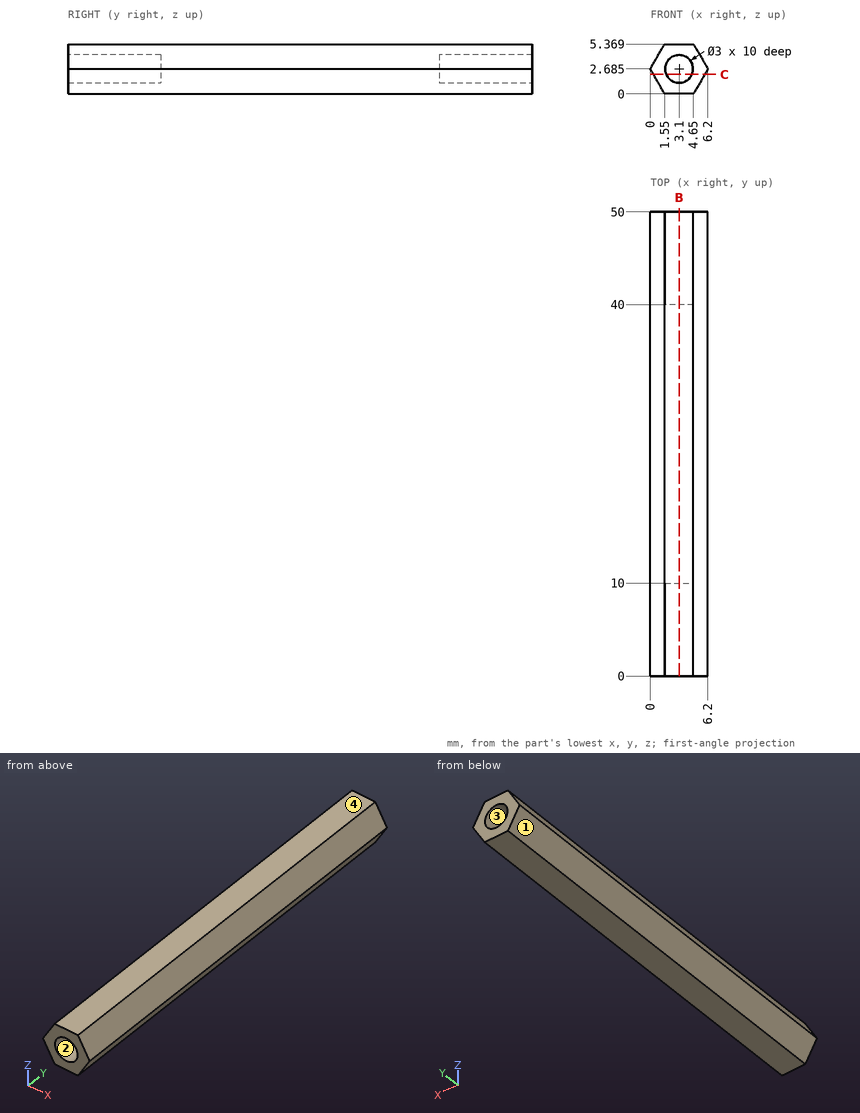
Geometry: see drawing. Coordinates: mm, zero at the bounding-box minimum. Give positions to 0.01 mm unless a question says otherwise; leave off trailing zeros. Loops run counter-clockwise (first coordinate to the right, second up) from the corner with the lowest first, then second, coordinate; pieces in that order, holes last. Notation, with made-up numbers: (58, 28) -> (72, 28) arc R9 ccw to (72, 35) -> close; hole circle Ø2 at (42.25, 34.5). An arc over 180 degrees is marked (long way). Answer as a JSON object with one key per item and string values. Group by question number.
Item 1: Pin query (flat end, axial travel): P1, Ø2, axis at y = 6.5, z = 0.5, coming from the +X side. Return the tip coordinate at first contact, or that it passes through.
Item 2: Pull-direction query (X, two-part tool) for the marked faces 1, 2, 3 and 4; classes: released by +X, released by -X, zero draft, split by the parting line, or undercut.
Item 3: Line query: probe 1 along Y at (x, z) = (3.25, 1.5); probe 2 along X at (y, z) = (38.5, 0.55); probe 3 along X at (y, z) = (3, 4.85). Output: solid intervals per line, ascending.
Item 4: Cut plane C-C, the plane z = 2.1. Return the cut outline in (x, y), and give its area (3 significant figures).
Item 5: Cut plane B-B, the plane x = 3.1. Return the cut outline in (y, z) (1 decimal).
Checks:
{
 "1": {"P1": "stops at x = 5.52"},
 "2": {"face 1": "released by -X", "face 2": "undercut", "face 3": "undercut", "face 4": "zero draft"},
 "3": {"probe 1": "y = 10 to 40", "probe 2": "x = 1.23 to 4.97", "probe 3": "x = 1.25 to 4.95"},
 "4": {"outline": "(0.34, 0) -> (1.72, 0) -> (1.72, 10) -> (4.48, 10) -> (4.48, 0) -> (5.86, 0) -> (5.86, 50) -> (4.48, 50) -> (4.48, 40) -> (1.72, 40) -> (1.72, 50) -> (0.34, 50) -> close", "area": "221 mm²"},
 "5": {"outline": "(0, 0) -> (50, 0) -> (50, 1.2) -> (40, 1.2) -> (40, 4.2) -> (50, 4.2) -> (50, 5.4) -> (0, 5.4) -> (0, 4.2) -> (10, 4.2) -> (10, 1.2) -> (0, 1.2) -> close"}
}
